from build123d import *

# Parameters (mm, degrees)
SKETCH1_W           = 124
SKETCH1_H           = 184
SKETCH1_R           = 2.5
BOSS_EXTRUDE1_DEPTH = 2
CUT_EXTRUDE2_REACH  = 112.959
SKETCH5_R           = 4.6


with BuildPart() as part:
    # Sketch1 → Boss-Extrude1 (new body)
    with BuildSketch(Plane(origin=(0, 60, 0), x_dir=(1, 0, 0), z_dir=(0, 1, 0))):
        Rectangle(SKETCH1_W, SKETCH1_H)
        with Locations(Location((-40.132, 79.51715957, 0), (0, 0, 270))):
            Circle(SKETCH1_R, mode=Mode.SUBTRACT)
        with Locations(Location((-20.066, 79.51715957, 0), (0, 0, 270))):
            Circle(SKETCH1_R, mode=Mode.SUBTRACT)
        with Locations(Location((0, 79.51715957, 0), (0, 0, 270))):
            Circle(SKETCH1_R, mode=Mode.SUBTRACT)
        with Locations(Location((20.066, 79.51715957, 0), (0, 0, 270))):
            Circle(SKETCH1_R, mode=Mode.SUBTRACT)
        with Locations(Location((40.132, 79.51715957, 0), (0, 0, 270))):
            Circle(SKETCH1_R, mode=Mode.SUBTRACT)
        with Locations(Location((-20.066, 73.42115957, 0), (0, 0, 270))):
            Circle(SKETCH1_R, mode=Mode.SUBTRACT)
        with Locations(Location((0, 73.42115957, 0), (0, 0, 270))):
            Circle(SKETCH1_R, mode=Mode.SUBTRACT)
        with Locations(Location((20.066, 73.42115957, 0), (0, 0, 270))):
            Circle(SKETCH1_R, mode=Mode.SUBTRACT)
        with Locations(Location((40.132, 73.42115957, 0), (0, 0, 270))):
            Circle(SKETCH1_R, mode=Mode.SUBTRACT)
        with Locations(Location((-20.066, 67.32515957, 0), (0, 0, 270))):
            Circle(SKETCH1_R, mode=Mode.SUBTRACT)
        with Locations(Location((0, 67.32515957, 0), (0, 0, 270))):
            Circle(SKETCH1_R, mode=Mode.SUBTRACT)
        with Locations(Location((20.066, 67.32515957, 0), (0, 0, 270))):
            Circle(SKETCH1_R, mode=Mode.SUBTRACT)
        with Locations(Location((40.132, 67.32515957, 0), (0, 0, 270))):
            Circle(SKETCH1_R, mode=Mode.SUBTRACT)
        with Locations(Location((-20.066, 61.22915957, 0), (0, 0, 270))):
            Circle(SKETCH1_R, mode=Mode.SUBTRACT)
        with Locations(Location((0, 61.22915957, 0), (0, 0, 270))):
            Circle(SKETCH1_R, mode=Mode.SUBTRACT)
        with Locations(Location((20.066, 61.22915957, 0), (0, 0, 270))):
            Circle(SKETCH1_R, mode=Mode.SUBTRACT)
        with Locations(Location((40.132, 61.22915957, 0), (0, 0, 270))):
            Circle(SKETCH1_R, mode=Mode.SUBTRACT)
        with Locations(Location((-20.066, 55.13315957, 0), (0, 0, 270))):
            Circle(SKETCH1_R, mode=Mode.SUBTRACT)
        with Locations(Location((0, 55.13315957, 0), (0, 0, 270))):
            Circle(SKETCH1_R, mode=Mode.SUBTRACT)
        with Locations(Location((20.066, 55.13315957, 0), (0, 0, 270))):
            Circle(SKETCH1_R, mode=Mode.SUBTRACT)
        with Locations(Location((40.132, 55.13315957, 0), (0, 0, 270))):
            Circle(SKETCH1_R, mode=Mode.SUBTRACT)
        with Locations(Location((-20.066, 49.03715957, 0), (0, 0, 270))):
            Circle(SKETCH1_R, mode=Mode.SUBTRACT)
        with Locations(Location((0, 49.03715957, 0), (0, 0, 270))):
            Circle(SKETCH1_R, mode=Mode.SUBTRACT)
        with Locations(Location((20.066, 49.03715957, 0), (0, 0, 270))):
            Circle(SKETCH1_R, mode=Mode.SUBTRACT)
        with Locations(Location((40.132, 49.03715957, 0), (0, 0, 270))):
            Circle(SKETCH1_R, mode=Mode.SUBTRACT)
        with Locations(Location((-20.066, 42.94115957, 0), (0, 0, 270))):
            Circle(SKETCH1_R, mode=Mode.SUBTRACT)
        with Locations(Location((0, 42.94115957, 0), (0, 0, 270))):
            Circle(SKETCH1_R, mode=Mode.SUBTRACT)
        with Locations(Location((20.066, 42.94115957, 0), (0, 0, 270))):
            Circle(SKETCH1_R, mode=Mode.SUBTRACT)
        with Locations(Location((40.132, 42.94115957, 0), (0, 0, 270))):
            Circle(SKETCH1_R, mode=Mode.SUBTRACT)
        with Locations(Location((-20.066, 36.84515957, 0), (0, 0, 270))):
            Circle(SKETCH1_R, mode=Mode.SUBTRACT)
        with Locations(Location((0, 36.84515957, 0), (0, 0, 270))):
            Circle(SKETCH1_R, mode=Mode.SUBTRACT)
        with Locations(Location((20.066, 36.84515957, 0), (0, 0, 270))):
            Circle(SKETCH1_R, mode=Mode.SUBTRACT)
        with Locations(Location((40.132, 36.84515957, 0), (0, 0, 270))):
            Circle(SKETCH1_R, mode=Mode.SUBTRACT)
        with Locations(Location((-20.066, 30.74915957, 0), (0, 0, 270))):
            Circle(SKETCH1_R, mode=Mode.SUBTRACT)
        with Locations(Location((0, 30.74915957, 0), (0, 0, 270))):
            Circle(SKETCH1_R, mode=Mode.SUBTRACT)
        with Locations(Location((20.066, 30.74915957, 0), (0, 0, 270))):
            Circle(SKETCH1_R, mode=Mode.SUBTRACT)
        with Locations(Location((40.132, 30.74915957, 0), (0, 0, 270))):
            Circle(SKETCH1_R, mode=Mode.SUBTRACT)
        with Locations(Location((-20.066, 24.65315957, 0), (0, 0, 270))):
            Circle(SKETCH1_R, mode=Mode.SUBTRACT)
        with Locations(Location((0, 24.65315957, 0), (0, 0, 270))):
            Circle(SKETCH1_R, mode=Mode.SUBTRACT)
        with Locations(Location((20.066, 24.65315957, 0), (0, 0, 270))):
            Circle(SKETCH1_R, mode=Mode.SUBTRACT)
        with Locations(Location((40.132, 24.65315957, 0), (0, 0, 270))):
            Circle(SKETCH1_R, mode=Mode.SUBTRACT)
        with Locations(Location((-40.132, 73.42115957, 0), (0, 0, 270))):
            Circle(SKETCH1_R, mode=Mode.SUBTRACT)
        with Locations(Location((-40.132, 67.32515957, 0), (0, 0, 270))):
            Circle(SKETCH1_R, mode=Mode.SUBTRACT)
        with Locations(Location((-40.132, 61.22915957, 0), (0, 0, 270))):
            Circle(SKETCH1_R, mode=Mode.SUBTRACT)
        with Locations(Location((-40.132, 55.13315957, 0), (0, 0, 270))):
            Circle(SKETCH1_R, mode=Mode.SUBTRACT)
        with Locations(Location((-40.132, 49.03715957, 0), (0, 0, 270))):
            Circle(SKETCH1_R, mode=Mode.SUBTRACT)
        with Locations(Location((-40.132, 42.94115957, 0), (0, 0, 270))):
            Circle(SKETCH1_R, mode=Mode.SUBTRACT)
        with Locations(Location((-40.132, 36.84515957, 0), (0, 0, 270))):
            Circle(SKETCH1_R, mode=Mode.SUBTRACT)
        with Locations(Location((-40.132, 30.74915957, 0), (0, 0, 270))):
            Circle(SKETCH1_R, mode=Mode.SUBTRACT)
        with Locations(Location((-40.132, 24.65315957, 0), (0, 0, 270))):
            Circle(SKETCH1_R, mode=Mode.SUBTRACT)
    extrude(amount=BOSS_EXTRUDE1_DEPTH)

    # Sketch5 → Cut-Extrude2 (cut, up to next)
    with BuildSketch(Plane(origin=(0, 62, 0), x_dir=(1, 0, 0), z_dir=(0, 1, 0)), mode=Mode.PRIVATE) as cut_extrude2_sk1:
        with Locations(Location((-44.45, -67, 0), (0, 0, 270))):
            Circle(SKETCH5_R)
    cut_extrude2_tool1 = extrude(cut_extrude2_sk1.sketch, amount=-CUT_EXTRUDE2_REACH, mode=Mode.PRIVATE) & part.part
    # Sketch5 → Cut-Extrude2 (cut, up to next)
    with BuildSketch(Plane(origin=(0, 62, 0), x_dir=(1, 0, 0), z_dir=(0, 1, 0)), mode=Mode.PRIVATE) as cut_extrude2_sk2:
        with Locations(Location((-26.67, -67, 0), (0, 0, 270))):
            Circle(SKETCH5_R)
    cut_extrude2_tool2 = extrude(cut_extrude2_sk2.sketch, amount=-CUT_EXTRUDE2_REACH, mode=Mode.PRIVATE) & part.part
    # Sketch5 → Cut-Extrude2 (cut, up to next)
    with BuildSketch(Plane(origin=(0, 62, 0), x_dir=(1, 0, 0), z_dir=(0, 1, 0)), mode=Mode.PRIVATE) as cut_extrude2_sk3:
        with Locations(Location((-8.89, -67, 0), (0, 0, 270))):
            Circle(SKETCH5_R)
    cut_extrude2_tool3 = extrude(cut_extrude2_sk3.sketch, amount=-CUT_EXTRUDE2_REACH, mode=Mode.PRIVATE) & part.part
    # Sketch5 → Cut-Extrude2 (cut, up to next)
    with BuildSketch(Plane(origin=(0, 62, 0), x_dir=(1, 0, 0), z_dir=(0, 1, 0)), mode=Mode.PRIVATE) as cut_extrude2_sk4:
        with Locations(Location((8.89, -67, 0), (0, 0, 270))):
            Circle(SKETCH5_R)
    cut_extrude2_tool4 = extrude(cut_extrude2_sk4.sketch, amount=-CUT_EXTRUDE2_REACH, mode=Mode.PRIVATE) & part.part
    # Sketch5 → Cut-Extrude2 (cut, up to next)
    with BuildSketch(Plane(origin=(0, 62, 0), x_dir=(1, 0, 0), z_dir=(0, 1, 0)), mode=Mode.PRIVATE) as cut_extrude2_sk5:
        with Locations(Location((26.67, -67, 0), (0, 0, 270))):
            Circle(SKETCH5_R)
    cut_extrude2_tool5 = extrude(cut_extrude2_sk5.sketch, amount=-CUT_EXTRUDE2_REACH, mode=Mode.PRIVATE) & part.part
    # Sketch5 → Cut-Extrude2 (cut, up to next)
    with BuildSketch(Plane(origin=(0, 62, 0), x_dir=(1, 0, 0), z_dir=(0, 1, 0)), mode=Mode.PRIVATE) as cut_extrude2_sk6:
        with Locations(Location((44.45, -67, 0), (0, 0, 270))):
            Circle(SKETCH5_R)
    cut_extrude2_tool6 = extrude(cut_extrude2_sk6.sketch, amount=-CUT_EXTRUDE2_REACH, mode=Mode.PRIVATE) & part.part
    add(cut_extrude2_tool1.solids().sort_by_distance((-44.45, 62, 67))[0], mode=Mode.SUBTRACT)
    add(cut_extrude2_tool2.solids().sort_by_distance((-26.67, 62, 67))[0], mode=Mode.SUBTRACT)
    add(cut_extrude2_tool3.solids().sort_by_distance((-8.89, 62, 67))[0], mode=Mode.SUBTRACT)
    add(cut_extrude2_tool4.solids().sort_by_distance((8.89, 62, 67))[0], mode=Mode.SUBTRACT)
    add(cut_extrude2_tool5.solids().sort_by_distance((26.67, 62, 67))[0], mode=Mode.SUBTRACT)
    add(cut_extrude2_tool6.solids().sort_by_distance((44.45, 62, 67))[0], mode=Mode.SUBTRACT)


solid = part.part
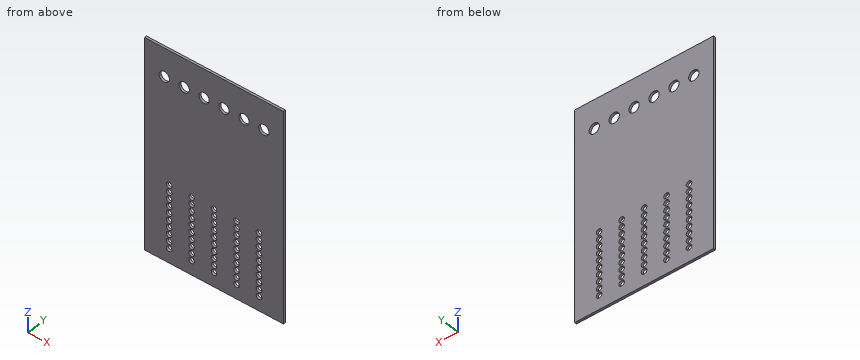
CAD build for the part. Positions are in the model's coordinates, mm. Round coordinates to 2 decimals unless told otherwise and drop trailing zeros. Write each loop counter-clockwise with the first axis right and the second up, starting at its lowest first coordinate (ties: lowest second). Pieces come first, ordered by that corner, then holes. Notation, with made-up numbers: M -1.5,77 L 41.5,77 A21 ccw 41.5,102 Z; hole C 6.25,68 d11. An arc over 180 degrees is marked long. Put each result on its own line as item: value. Start each with the question number.
1) Saw through at C-C, the plane y = 60.9. Count the separate pieces of the cut face and the enclosed holes in it, and give its area (3 significant figures).
2) Saw through at B-B, the plane x = -11. Write the cut outline in (y, z), and give its area (3 significant figures).
3) Drill centre lines: probe 1 along X at (y, z) = (60.6, -36); probe 2 along X at (y, z) = (60.5, -47.5); probe 3 along Z at (x, y) = (27, 60.7). Where is each one in solid material? Low to high. Write a range as [from, to].
4) Saw through at A-A, the plane x = 26.67. Write the cut outline in (y, z), and give its area (3 significant figures).
Resolved:
1. separate pieces: 1
1. enclosed holes: 56
1. area: 21,400 mm²
2. outline: M 60,-92 L 62,-92 L 62,62.91 L 60,62.91 Z; M 60,71.09 L 62,71.09 L 62,92 L 60,92 Z
2. area: 352 mm²
3. probe 1: [-62, -42.48], [-37.78, -22.42], [-17.71, -2.35], [2.35, 17.71], [22.42, 37.78], [42.48, 62]
3. probe 2: [-62, -42.1], [-38.16, -22.04], [-18.09, -1.97], [1.97, 18.09], [22.04, 38.16], [42.1, 62]
3. probe 3: [-92, 62.41], [71.59, 92]
4. outline: M 60,-92 L 62,-92 L 62,62.4 L 60,62.4 Z; M 60,71.6 L 62,71.6 L 62,92 L 60,92 Z
4. area: 350 mm²
